from build123d import *

# Parameters (mm, degrees)
BOSS_EXTRUDE1_DEPTH = 38.1
SHELL1_T            = -3.175
SKETCH4_R           = 15.875
BOSS_EXTRUDE3_DEPTH = 28.575
BOSS_EXTRUDE4_DEPTH = 28.575
SKETCH6_R           = 15.875
CUT_EXTRUDE2_DEPTH  = 25.4
CUT_EXTRUDE3_START  = 25.4
SKETCH6_2_R         = 15.875
CUT_EXTRUDE3_DEPTH  = 25.4
CUT_EXTRUDE4_REACH  = 109.606
SKETCH7_R           = 3.175
BOSS_EXTRUDE5_REACH = 109.606
CUT_EXTRUDE5_DEPTH  = 25.4


with BuildPart() as part:
    # Sketch2 → Boss-Extrude1 (new, symmetric)
    with BuildSketch(Plane(origin=(0, 0, 0), x_dir=(0, 0, -1), z_dir=(1, 0, 0))):
        with BuildLine():
            Line((0, 0), (53.881536726, 53.881536726))
            ThreePointArc((53.881536726, 53.881536726), (0, 53.881536726), (0, 0))
        make_face()
    extrude(amount=BOSS_EXTRUDE1_DEPTH, both=True)

    # Shell1
    shell1_openings = [part.faces().sort_by_distance(p)[0] for p in [
        (0, 26.940768363, -26.940768363),
    ]]
    offset(amount=SHELL1_T, openings=shell1_openings)

    # Chamfer1
    # the kernel refuses this chamfer: 10 mm, written as the material it takes off along each edge
    with BuildSketch(Plane(origin=(34.925, 51.636472696, -51.636472696), x_dir=(0, 0.6876558872178, -0.726036762688158), z_dir=(-1, 0, 0))) as chamfer1_piece_1:
        with BuildLine():
            Line((8.869626963, -0.240804851), (-1.086879529, -7.747424349))
            ThreePointArc((-1.086879529, -7.747424349), (-0.345966855, -4.045712731), (0, 0))
            Line((0, 0), (8.869626963, -0.240804851))
        make_face()
    extrude(amount=69.85, mode=Mode.SUBTRACT)



with BuildPart() as body_2:
    # Sketch4 → Boss-Extrude3 (new, symmetric)
    with BuildSketch(Plane(origin=(0, 0, 0), x_dir=(0, 0, -1), z_dir=(1, 0, 0))):
        with Locations((0, -15.875)):
            Circle(SKETCH4_R)
    extrude(amount=BOSS_EXTRUDE3_DEPTH, both=True)


with BuildPart() as part_1:
    add(part.part)

    add(body_2.part)  # Boss-Extrude4 merges body 2
    # Sketch5 → Boss-Extrude4 (add, symmetric)
    with BuildSketch(Plane(origin=(0, 0, 0), x_dir=(0, 0, -1), z_dir=(1, 0, 0))):
        Polygon((2.24506403, 2.24506403), (2.24506403, -0.159551788), (0, 0), align=None)
    extrude(amount=BOSS_EXTRUDE4_DEPTH, both=True)

    # Sketch6 → Cut-Extrude2 (cut)
    with BuildSketch(Plane(origin=(0, 0, 0), x_dir=(0, 0, -1), z_dir=(1, 0, 0))):
        with Locations((0, -15.875)):
            Circle(SKETCH6_R)
    extrude(amount=-CUT_EXTRUDE2_DEPTH, mode=Mode.SUBTRACT)

    # Sketch6<2> → Cut-Extrude3 (cut)
    with BuildSketch(Plane(origin=(0, 0, 0), x_dir=(0, 0, -1), z_dir=(1, 0, 0)).offset(CUT_EXTRUDE3_START)):
        with Locations((0, -15.875)):
            Circle(SKETCH6_2_R)
    extrude(amount=-CUT_EXTRUDE3_DEPTH, mode=Mode.SUBTRACT)

    # Cut-Extrude4: up to this face of the body (flat: up to its plane)
    cut_extrude4_end = Plane(part_1.part.faces().sort_by_distance((28.575, -15.819887854, -0.005001009))[0])
    # Sketch7 → Cut-Extrude4 (cut, up to the picked face)
    with BuildSketch(Plane.ZY.offset(28.575), mode=Mode.PRIVATE) as cut_extrude4_sk1:
        with Locations(Location((0, -15.875, 0), (0, 0, 180))):
            Circle(SKETCH7_R)
    cut_extrude4_tool1 = split(extrude(cut_extrude4_sk1.sketch, amount=-CUT_EXTRUDE4_REACH, mode=Mode.PRIVATE), bisect_by=cut_extrude4_end, keep=Keep.BOTH, mode=Mode.PRIVATE)
    add(cut_extrude4_tool1.solids().sort_by(Axis((-28.575, -15.875, 0), (1, 0, 0)))[0], mode=Mode.SUBTRACT)

    # Boss-Extrude5: up to this face of the body (flat: up to its plane)
    boss_extrude5_end = Plane(part_1.part.faces().sort_by_distance((-28.575, 0.79361509, -1.451448941))[0])
    # Sketch8 → Boss-Extrude5 (add, up to the picked face)
    with BuildSketch(Plane(origin=(28.575, 0, 0), x_dir=(0, 0, -1), z_dir=(1, 0, 0)), mode=Mode.PRIVATE) as boss_extrude5_sk1:
        with BuildLine():
            Line((-11.159231637, 26.940768363), (-15.875, -15.875))
            Line((-15.875, -15.875), (2.24506403, 2.24506403))
            ThreePointArc((2.24506403, 2.24506403), (-3.75420071, 10.280201189), (-7.223023717, 19.688807544))
            Line((-7.223023717, 19.688807544), (-11.159231637, 26.940768363))
        make_face()
    boss_extrude5_tool1 = split(extrude(boss_extrude5_sk1.sketch, amount=-BOSS_EXTRUDE5_REACH, mode=Mode.PRIVATE), bisect_by=boss_extrude5_end, keep=Keep.BOTH, mode=Mode.PRIVATE)
    add(boss_extrude5_tool1.solids().sort_by(Axis((28.575, 4.070009, 8.572047), (-1, 0, 0)))[0])

    # Sketch9 → Cut-Extrude5 (cut, symmetric)
    with BuildSketch(Plane(origin=(0, 0, 0), x_dir=(0, 0, -1), z_dir=(1, 0, 0))):
        with BuildLine():
            Line((2.24506403, -0.159551788), (2.24506403, 2.24506403))
            Line((2.24506403, 2.24506403), (0, 0))
            ThreePointArc((0, 0), (-8.259041825, 12.36052959), (-11.159231637, 26.940768363))
            Line((-11.159231637, 26.940768363), (-15.494456387, -12.419939034))
            ThreePointArc((-15.494456387, -12.419939034), (9.025844742, -28.934469809), (2.24506403, -0.159551788))
        make_face()
    extrude(amount=CUT_EXTRUDE5_DEPTH, both=True, mode=Mode.SUBTRACT)


solid = part_1.part
For this review, take the finished solid that the model builds, in its own axes (mm). A direction names the side the tool comes from. Round coordinates to 2 decimals unless told otherwise and drop trailing zeros. Write each loop counter-clockwise with the first axis right and the second up, starting at its lowest first coordinate (ties: lowest second). Pieces come first, ordered by that corner, then holes. Notation, with made-up numbers: (22, 76) - (39, 76) arc R31 ccw to (39, 105) - close; hole circle Ø6 at (86.5, -32.75). An arc over 180 degrees is marked (long way). Write item = value, one per line. Start each with the question number.
1. Consider section D-D on y = 18.5. State the section outline as (x, z) points (3 decimals), plus the area to 3 significant figures.
2. For pin 1 Ø1 at (x, y) = (12.5, 25.5) entering from -Z; pin 2 Ø10 at (y, z) = (-15.875, 0) entering from +X (3 decimals); pin 3 Ø3 at (x, y) = (-20.5, 23.5) entering from -Z, all flat-tipped, find the tip position at first contact; note any pin that passes through.
3. Draft analysis for pull direction X (two halves, no side actions). For faces 4 (the face through (0.489, 49.268, -0.085)), 5 (the face through (-27, 7.5, 13.3)), 6 (the face through (-28.575, -15, 3.3)), state which applies: released by +X, released by -X, zero draft, split by the parting line, or undercut.
4. Consider section A-A on y = 59. State the section outline as (x, z) points (3 decimals), plus the area to 3 significant figures.
5. For faces 1 (the face through (27, 1, -2.245)), 2 (the face through (27, 7.5, 13.3)), 3 (the face through (0.489, 56.786, -47.936)), list the 3-axis set-ups (+Z, -Z, +X, -X, +Y, -Y) from which the entire face can be reached by the end or side of a thin tool; tool diameter is ignored.
6. Consider section B-B on x = 2. State the section outline as (y, z) points (3 decimals).
7. Consider section C-C on y = 45. State the section outline as (x, z) points (3 decimals).
8. Wall thickness on L1, parallel to Y at x = 27.85, z = 0; L2, parallel to X at y = 16, z = 6 (3 decimals); L3, parallel to X at y = -1, z = 10 (3 decimals): over which ranges is each line inside the solid? List them lowest first.
Evaluation:
q1.outline = (-38.1, -18.5) - (-34.925, -18.5) - (-34.925, 6.949) - (34.925, 6.949) - (34.925, -18.5) - (38.1, -18.5) - (38.1, 10.212) - (28.575, 10.212) - (28.575, 12.089) - (25.4, 12.089) - (25.4, 10.212) - (-25.4, 10.212) - (-25.4, 12.089) - (-28.575, 12.089) - (-28.575, 10.212) - (-38.1, 10.212) - close
q1.area = 422 mm2
q2.pin_1 = 7.93
q2.pin_2 = 28.575
q2.pin_3 = 7.63
q3.face_4 = undercut
q3.face_5 = zero draft
q3.face_6 = released by -X
q4.outline = (-38.1, -47.528) - (38.1, -47.528) - (38.1, -6.354) - (-38.1, -6.354) - close; hole (-34.925, -40.796) - (34.925, -40.796) - (34.925, -13.086) - (-34.925, -13.086) - close
q4.area = 1,200 mm2
q5.face_1 = -Z, +X, -X
q5.face_2 = +Z, +X, -X, +Y
q5.face_3 = -Z, -Y
q6.outline = (0, 0) - (2.245, -2.245) arc R34.925 cw to (56.514, -45.52) - (57.051, -50.285) arc R38.1 ccw to start
q7.outline = (-38.1, -45) - (-34.925, -45) - (-34.925, 2.953) - (34.925, 2.953) - (34.925, -45) - (38.1, -45) - (38.1, 6.607) - (-38.1, 6.607) - close
q8.L1 = -31.75 to -19.05, -12.7 to 4.72, 49.17 to 53.88
q8.L2 = -38.1 to -34.925, 34.925 to 38.1
q8.L3 = -28.575 to -25.4, 25.4 to 28.575
